Geometry check sheet. Reference: the model listing, model coordinates, mm. A direction names the side the tool comes from. Give positions to 0.01 mm unless a question says otherwise; leave off trailing zeros.
```python
from build123d import *

# Parameters (mm, degrees)
SKETCH2_W           = 325
SKETCH2_H           = 225
SKETCH4_W           = 265
SKETCH4_H           = 165
SKETCH8_W           = 255
SKETCH8_H           = 155
SKETCH9_W           = 255
SKETCH9_H           = 155
SKETCH10_W          = 265
SKETCH10_H          = 165
BOSS_EXTRUDE1_DEPTH = 5
SKETCH13_W          = 10
SKETCH13_H          = 10
BOSS_EXTRUDE2_DEPTH = 162
SKETCH14_R          = 2.5
CUT_EXTRUDE1_DEPTH  = 196.0000001
CUT_EXTRUDE2_REACH  = 327
SKETCH15_W          = 15
SKETCH15_H          = 20


with BuildPart() as part:
    # Sketch2 → Loft2 section 0
    with BuildSketch(Plane(origin=(0, 0, 0), x_dir=(1, 0, 0), z_dir=(0, 1, 0))):
        with Locations((127.5, 77.5)):
            Rectangle(SKETCH2_W, SKETCH2_H)
    # Sketch4 → Loft2 section 1
    with BuildSketch(Plane(origin=(0, 190, 0), x_dir=(1, 0, 0), z_dir=(0, 1, 0))):
        with Locations((127.5, 77.5)):
            Rectangle(SKETCH4_W, SKETCH4_H)
    loft()

    # Sketch8 → Cut-Loft1 section 0
    with BuildSketch(Plane(origin=(0, 190, 0), x_dir=(1, 0, 0), z_dir=(0, 1, 0))):
        with Locations((127.5, 77.5)):
            Rectangle(SKETCH8_W, SKETCH8_H)
    # Sketch9 → Cut-Loft1 section 1
    with BuildSketch(Plane.XZ):
        with Locations((127.5, -77.5)):
            Rectangle(SKETCH9_W, SKETCH9_H)
    loft(mode=Mode.SUBTRACT)

    # Sketch10 → Boss-Extrude1 (add)
    with BuildSketch(Plane(origin=(0, 190, 0), x_dir=(1, 0, 0), z_dir=(0, 1, 0))):
        with Locations((127.5, 77.5)):
            Rectangle(SKETCH10_W, SKETCH10_H)
    extrude(amount=BOSS_EXTRUDE1_DEPTH)

    # Sketch13 → Boss-Extrude2 (add)
    with BuildSketch(Plane(origin=(0, 33, 0), x_dir=(1, 0, 0), z_dir=(0, 1, 0))):
        with Locations((5, 150)):
            Rectangle(SKETCH13_W, SKETCH13_H)
        with Locations((250, 150)):
            Rectangle(SKETCH13_W, SKETCH13_H)
        with Locations((250, 5)):
            Rectangle(SKETCH13_W, SKETCH13_H)
        with Locations((5, 5)):
            Rectangle(SKETCH13_W, SKETCH13_H)
    extrude(amount=BOSS_EXTRUDE2_DEPTH)

    # Sketch14 → Cut-Extrude1 (cut, through all)
    with BuildSketch(Plane(origin=(0, 195, 0), x_dir=(1, 0, 0), z_dir=(0, 1, 0))):
        with Locations((65, 47.5)):
            Circle(SKETCH14_R)
        with Locations((65, 67.5)):
            Circle(SKETCH14_R)
        with Locations((95, 67.5)):
            Circle(SKETCH14_R)
        with Locations((95, 47.5)):
            Circle(SKETCH14_R)
        with Locations((95, 107.5)):
            Circle(SKETCH14_R)
        with Locations((95, 87.5)):
            Circle(SKETCH14_R)
        with Locations((65, 87.5)):
            Circle(SKETCH14_R)
        with Locations((65, 107.5)):
            Circle(SKETCH14_R)
    extrude(amount=-CUT_EXTRUDE1_DEPTH, mode=Mode.SUBTRACT)

    # Sketch15 → Cut-Extrude2 (cut, up to next)
    with BuildSketch(Plane(origin=(290, 0, 0), x_dir=(0, 0, -1), z_dir=(1, 0, 0)), mode=Mode.PRIVATE) as cut_extrude2_sk1:
        with Locations((22.5, 60)):
            Rectangle(SKETCH15_W, SKETCH15_H)
    cut_extrude2_tool1 = extrude(cut_extrude2_sk1.sketch, amount=-CUT_EXTRUDE2_REACH, mode=Mode.PRIVATE) & part.part
    add(cut_extrude2_tool1.solids().sort_by_distance((290, 60, -22.5))[0], mode=Mode.SUBTRACT)
    # Sketch15 → Cut-Extrude2 (cut, up to next)
    with BuildSketch(Plane(origin=(290, 0, 0), x_dir=(0, 0, -1), z_dir=(1, 0, 0)), mode=Mode.PRIVATE) as cut_extrude2_sk2:
        with Locations((132.5, 60)):
            Rectangle(SKETCH15_W, SKETCH15_H)
    cut_extrude2_tool2 = extrude(cut_extrude2_sk2.sketch, amount=-CUT_EXTRUDE2_REACH, mode=Mode.PRIVATE) & part.part
    add(cut_extrude2_tool2.solids().sort_by_distance((290, 60, -132.5))[0], mode=Mode.SUBTRACT)


solid = part.part
```
1) Depth check by flat-ended pin: P1, Ø8, axis at x = 249.5, z = -148.5, coming from the -Y side; P2, Ø5, axis at x = 81, y = 130, coming from the +Z side; P3, Ø16, axis at x = 272, y = 58.5, coming from the +Z side. Enter the tip coordinate at first touch or a pass-through.
2) Scan lines: line 1 along Z through (x, y) = (65, 191.4); line 2 along X through (y, z) = (192.7, -47.5); line 3 along Y through (x, z) = (6, -126.5). Record each from-to range of solid material in increasing order.
3) Mould release check, pull along X, two halves, no side actions. Record for faces 3 (the flat face through (245, 110, -150)), 4 (the flat face through (269, 50, -132)): +X half, -X half, draft (parallel to the pull), parting line (faces both ways), or undercut.
4) Tool access check on faces 1 (the flat face through (269, 60, -30)), 2 (the flat face through (5, 110, -10)). Record the directions out of +Z, -Z, +X, -X, +Y, -Y that give a thin tool (end or side, any length) a straight path to the whole face; none if there is none.
Determined:
1. P1: stops at y = 33
1. P2: stops at z = 14.87
1. P3: stops at z = 27.03
2. line 1: z = -160 to -110, -105 to -90, -85 to -70, -65 to -50, -45 to 5
2. line 2: x = -5 to 62.5, 67.5 to 92.5, 97.5 to 260
2. line 3: y = 190 to 195
3. face 3: undercut
3. face 4: draft
4. face 1: +X
4. face 2: -Y
